Could you check a few things on this drawing? It's one solid part, dimensions in mm from its lowest x, y, z. A direction names the side the tool comes from. Round coordinates to 2 decimals unless told otherwise and drop trailing zeros. Write each loop counter-clockwise with the first axis right and the second up, starting at its lowest first coordinate (ties: lowest second). Pieces come first, ordered by that corner, then holes. Notation, with made-up numbers: (20.25, 32) - (47.25, 32) arc R17 ccw to (47.25, 56) - close; hole circle Ø5 at (68, 86). An arc over 180 degrees is marked (long way). Use one line per item in the form item = value. Start each with the question number.
1. I want a section at A-A, the plane z = 48.95. List the corners of the cut face in (x, y) for me, plus the area to 3 significant figures.
2. Which directions (+Z, -Z, +X, -X, +Y, -Y) give clear straight access to the entire face, cutting with the end or side of a thin tool? Please do the marked faces 1, 2, 3, 4 and 5.
3. I want a section at B-B, the plane y = 30. List the corners of the cut face in (x, z) for me.
4. Will these pins go through, and if not, where does the flat tip stop? pin 1 (1 mm diameter, centred on y = 14.5, z = 45.5, fed in from -X); pin 2 (12.5 mm diameter, centred on x = 27.5, y = 10.5, fed in from -Z); pin 3 (3 mm diameter, centred on y = 23, z = 28, fed in from -X); pin 4 (2.5 mm diameter, centred on y = 33.37, z = 48.95, fed in from +X).
5. We'd pull the mould along Y, two halves only. Please class the marked faces 6, 7, 8 and 9: +Y half, -Y half, draft (parallel to the pull), parting line (faces both ways), or undercut.
6. If I drill on line 1 along Z through (x, y) = (38, 2); line 2 along X through (y, z) = (36, 47); line 3 along X through (y, z) = (1.4, 16.51), over which ranges is the centre line in solid material (lowest first)?
7. I want a section at D-D, the plane x = 11.43. List the corners of the cut face in (y, z) for me (1 decimal).
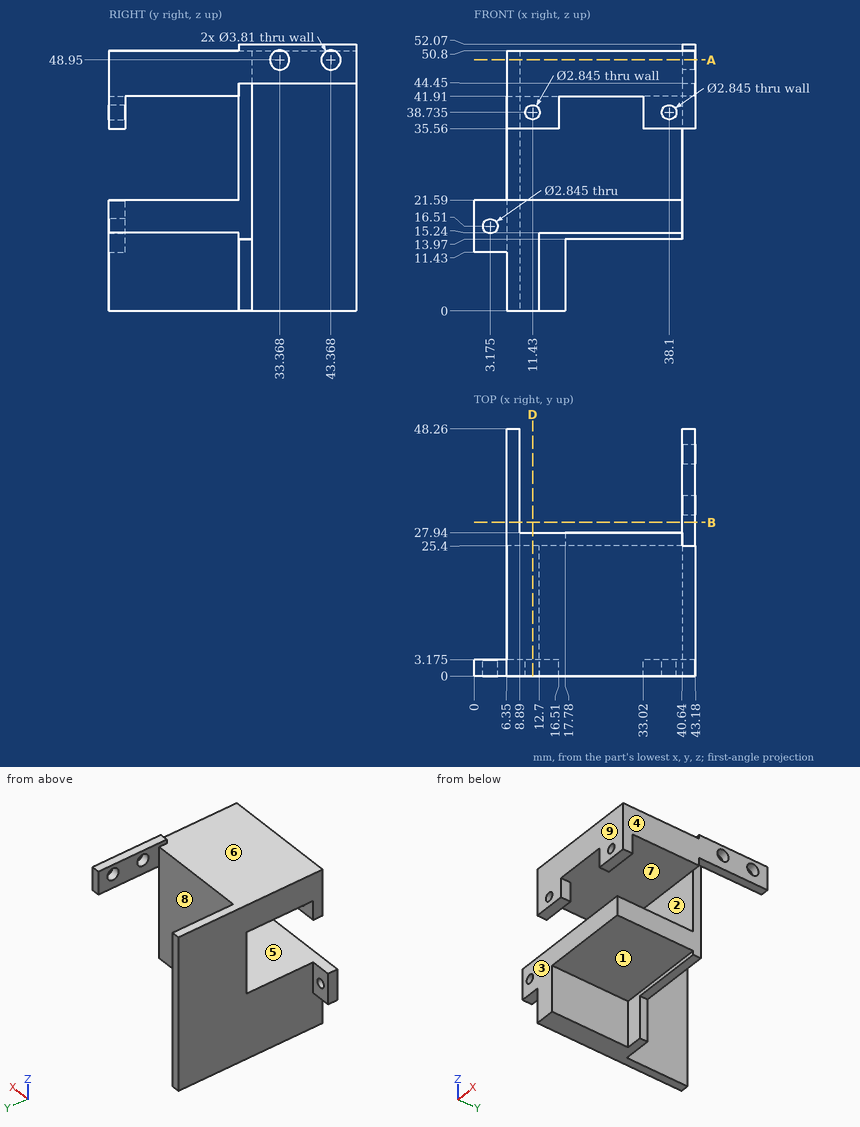
Model answer:
q1.outline = (6.35, 0) - (43.18, 0) - (43.18, 31.46) - (40.64, 31.46) - (40.64, 27.94) - (8.89, 27.94) - (8.89, 48.26) - (6.35, 48.26) - close; (40.64, 35.27) - (43.18, 35.27) - (43.18, 41.46) - (40.64, 41.46) - close; (40.64, 45.27) - (43.18, 45.27) - (43.18, 48.26) - (40.64, 48.26) - close
q1.area = 1,110 mm2
q2.face_1 = -Z, +X, -Y
q2.face_2 = +X, -X
q2.face_3 = +Z, -Z, +X, -X, -Y
q2.face_4 = +Z, -Z, +X, +Y, -Y
q2.face_5 = +X, -X, -Y
q3.outline = (6.35, 0) - (8.89, 0) - (8.89, 50.8) - (6.35, 50.8) - close; (40.64, 44.45) - (43.18, 44.45) - (43.18, 52.07) - (40.64, 52.07) - close
q4.pin_1 = 6.35
q4.pin_2 = 15.24
q4.pin_3 = through
q4.pin_4 = 8.89
q5.face_6 = draft
q5.face_7 = undercut
q5.face_8 = +Y half
q5.face_9 = -Y half
q6.line_1 = 15.24 to 21.59, 35.56 to 37.32, 40.15 to 50.8
q6.line_2 = 6.35 to 8.89, 40.64 to 43.18
q6.line_3 = 0 to 1.75, 4.6 to 40.64
q7.outline = (0, 0) - (27.9, 0) - (27.9, 50.8) - (0, 50.8) - (0, 40.2) - (3.2, 40.2) - (3.2, 41.9) - (25.4, 41.9) - (25.4, 21.6) - (0, 21.6) - close; (0, 35.6) - (3.2, 35.6) - (3.2, 37.3) - (0, 37.3) - close
